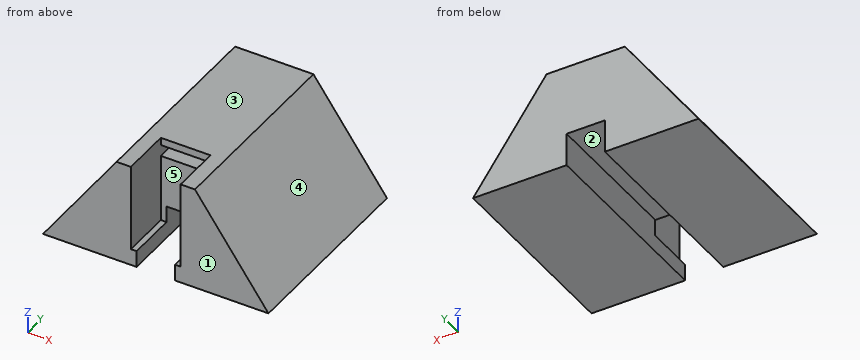
from build123d import *

# Parameters (mm, degrees)
F1_W      = 20.5
F1_H      = 51.5
F2_DEPTH  = 27.11
F4_W      = 59
F4_H      = 51.5
F3_W      = 20.5
F3_H      = 51.5
F6_W      = 10
F6_H      = 13
F7_DEPTH  = 27.11
F8_W      = 13
F8_H      = 13
F9_DEPTH  = 22.75
F10_W     = 10
F10_H     = 8.67
F11_DEPTH = 38.5
F12_W     = 13
F12_H     = 3
F13_DEPTH = 5


with BuildPart() as f2:
    # F1 (on face) → F2 (new body)
    with BuildSketch(Plane.XY):
        Rectangle(F1_W, F1_H)
    extrude(amount=F2_DEPTH)

    # F4 (on face) → F5 section 0
    with BuildSketch(Plane.XY):
        Rectangle(F4_W, F4_H)
    # F3 (on face) → F5 section 1
    with BuildSketch(Plane.XY.offset(27.11)):
        Rectangle(F3_W, F3_H)
    loft()

    # F6 (on face) → F7 (cut, through all)
    with BuildSketch(Plane.XY.offset(27.11)):
        with Locations((0, -19.25)):
            Rectangle(F6_W, F6_H)
    extrude(amount=-F7_DEPTH, mode=Mode.SUBTRACT)

    # F8 (on face) → F9 (cut)
    with BuildSketch(Plane.XY.offset(27.11)):
        with Locations((0, -19.25)):
            Rectangle(F8_W, F8_H)
    extrude(amount=-F9_DEPTH, mode=Mode.SUBTRACT)

    # F10 (on face) → F11 (cut, through all)
    with BuildSketch(Plane.XZ.offset(12.75)):
        with Locations((0, 4.335)):
            Rectangle(F10_W, F10_H)
    extrude(amount=-F11_DEPTH, mode=Mode.SUBTRACT)

    # F12 (on face) → F13 (cut)
    with BuildSketch(Plane.XZ.offset(12.75)):
        with Locations((0, 23.61)):
            Rectangle(F12_W, F12_H)
    extrude(amount=-F13_DEPTH, mode=Mode.SUBTRACT)


solid = f2.part
The model under review builds one solid part; all positions refer to its coordinate system, in mm. Face numbers are marked on the shaded views. A direction names the side the tool comes from. Give positions to 0.01 mm unless a question says otherwise; leave off trailing zeros. Loops run counter-clockwise (first coordinate to the right, second up) from the corner with the lowest first, then second, coordinate; pieces in that order, holes last. Notation, with made-up numbers: (-2, 77) -> (42, 77) arc R12 ccw to (42, 96) -> close; hole circle Ø9 at (-4.5, 80). An arc over 180 degrees is marked (long way). Answer as a JSON object with one key per item and string values. Group by question number.
Q1. Wall thickness on line 1 along Y through (x, z) = (4.5, 9.75); line 2 along X through (y, z) = (-20.5, 19.5); line 3 along X through (y, z) = (23.5, 6.25): over which ranges is each line inside the solid? List them lowest first.
Q2. Tool access review of the marked faces 1 and 2: name each direction out of +Z, -Z, +X, -X, +Y, -Y from which nothing blocks a thin tool from reaching the whole face with its end or side.
Q3. Draft analysis for pull direction X (two halves, no side actions). For the marked faces 3, 4 and 5, state which applies: pulls with the +X half, pulls with the -X half, needs draft (parallel to the pull), parting line crosses it, or undercut.
Q4. Insertion check: pin 1 (7 mm diameter, centred on y = -3, z = 5.5, fed in from +X); pin 2 (3 mm diameter, centred on x = -0.5, y = 12.5, fed in from -Z); pin 3 (1.2 mm diameter, centred on x = -6, y = -21, fed in from +Z); pin 4 (8 mm diameter, centred on y = -3, z = 23.5, fed in from -X). Each pin has a flat end and moves straight along its axis. Give the tip position at first contact, or say it passes through.
Q5. Take a section at C-C (x = 4). Write out the cut boundary in (y, z), plus the area to 3 significant figures.
Q6. Take a section at A-A (z = 6.5). Write out the cut boundary in (x, y).
Q7. Take a section at D-D (z = 2). Write out the cut boundary in (x, y).
Q8. Take a section at B-B (y = -6.5). Write out the cut boundary in (x, z).
Answer below:
{
 "1": {"line 1": "y = -12.75 to 25.75", "line 2": "x = -15.65 to -6.5, 6.5 to 15.65", "line 3": "x = -25.06 to -5, 5 to 25.06"},
 "2": {"face 1": "+Z, -Z, +X, -X, -Y", "face 2": "-Z, +Y, -Y"},
 "3": {"face 3": "needs draft", "face 4": "pulls with the +X half", "face 5": "undercut"},
 "4": {"pin 1": "stops at x = 28.08", "pin 2": "stops at z = 8.67", "pin 3": "stops at z = 27.11", "pin 4": "stops at x = -15.65"},
 "5": {"outline": "(-12.75, 8.67) -> (25.75, 8.67) -> (25.75, 27.11) -> (-12.75, 27.11) -> (-12.75, 25.11) -> (-7.75, 25.11) -> (-7.75, 22.11) -> (-12.75, 22.11) -> close", "area": "695 mm2"},
 "6": {"outline": "(-24.88, -25.75) -> (-6.5, -25.75) -> (-6.5, -12.75) -> (-5, -12.75) -> (-5, 25.75) -> (-24.88, 25.75) -> close; (5, -12.75) -> (6.5, -12.75) -> (6.5, -25.75) -> (24.88, -25.75) -> (24.88, 25.75) -> (5, 25.75) -> close"},
 "7": {"outline": "(-28.08, -25.75) -> (-5, -25.75) -> (-5, 25.75) -> (-28.08, 25.75) -> close; (5, -25.75) -> (28.08, -25.75) -> (28.08, 25.75) -> (5, 25.75) -> close"},
 "8": {"outline": "(-29.5, 0) -> (-5, 0) -> (-5, 8.67) -> (5, 8.67) -> (5, 0) -> (29.5, 0) -> (10.25, 27.11) -> (-10.25, 27.11) -> close"}
}
